Read the model definition and answer for the solid it produces. Units are mm, in the model's axes. A direction names the side the tool comes from. Give positions to 0.01 mm unless a question says otherwise; leave off trailing zeros. Write each loop counter-clockwise with the first axis right and the second up, starting at its lowest first coordinate (ties: lowest second). Pieces come first, ordered by that corner, then holes. Notation, with made-up numbers: (12.5, 80) - (70.5, 80) arc R19 cw to (70.5, 86) - close; hole circle Ø9 at (-29, 56.25). An arc over 180 degrees is marked (long way). Answer as CSV lines item,"result".
```python
from build123d import *

# Parameters (mm, degrees)
SKETCH1_R               = 10
BOSS_EXTRUDE1_DEPTH     = 10
BOSS_EXTRUDE2_DEPTH     = 110
CUT_EXTRUDE2_DEPTH      = 200.025801938
CUT_EXTRUDE2_DEPTH_BACK = 110


with BuildPart() as part:
    # Sketch1 → Boss-Extrude1 (new body)
    with BuildSketch(Plane(origin=(0, 0, 0), x_dir=(1, 0, 0), z_dir=(0, 1, 0))):
        Polygon((60, 0), (0, 0), (0, 80), (140, 80), align=None)
        with Locations(Location((40, 40, 0), (0, 0, 270))):
            Circle(SKETCH1_R, mode=Mode.SUBTRACT)
    extrude(amount=BOSS_EXTRUDE1_DEPTH)

    # Sketch1_3 → Boss-Extrude2 (add)
    with BuildSketch(Plane(origin=(0, 0, 0), x_dir=(1, 0, 0), z_dir=(0, 1, 0))):
        Polygon((140, 80), (154.142135624, 65.857864376), (74.142135624, -14.142135624), (60, 0), align=None)
    extrude(amount=BOSS_EXTRUDE2_DEPTH)

    # Sketch2 → Cut-Extrude2 (cut, two sides: drawn at the far end of the back side and taken through both)
    with BuildSketch(Plane(origin=(44.142135624, 0, 44.142135624), x_dir=(0.7071067811865461, 0, -0.707106781186549), z_dir=(0.707106781186549, 0, 0.7071067811865461)).offset(-CUT_EXTRUDE2_DEPTH_BACK)):
        with BuildLine():
            Line((42.426406871, 110), (42.426406871, 92.625413423))
            ThreePointArc((42.426406871, 92.625413423), (66.915884537, 104.857221881), (93.802749132, 110))
            Line((93.802749132, 110), (42.426406871, 110))
        make_face()
        with BuildLine():
            Line((155.563491861, 110), (104.1871496, 110))
            ThreePointArc((104.1871496, 110), (131.074014195, 104.857221881), (155.563491861, 92.625413423))
            Line((155.563491861, 92.625413423), (155.563491861, 110))
        make_face()
        with BuildLine():
            Line((58.994949366, 80), (42.426406871, 80))
            Line((42.426406871, 80), (42.426406871, 40))
            Line((42.426406871, 40), (58.994949366, 40))
            ThreePointArc((58.994949366, 40), (78.994949366, 60), (58.994949366, 80))
        make_face()
        with BuildLine():
            Line((155.563491861, 40), (155.563491861, 80))
            Line((155.563491861, 80), (138.994949366, 80))
            ThreePointArc((138.994949366, 80), (118.994949366, 60), (138.994949366, 40))
            Line((138.994949366, 40), (155.563491861, 40))
        make_face()
    extrude(amount=CUT_EXTRUDE2_DEPTH + CUT_EXTRUDE2_DEPTH_BACK, mode=Mode.SUBTRACT)


solid = part.part
```
(1) For faces 5 (the flat face through (141, 40, -67)), 6 (the flat face through (30, 5, 0)), 7 (the flat face through (73, 40, 1)), 8 (the flat face through (55, 10, -49)), 9 (the flat face through (69, 5, -80)), determine the directions among +Z, -Z, +X, -X, +Y, -Y from which every point of the face is accessible in a straight line to the end or side of a thin tool.
Worked out:
face 5,"-Z, +X"
face 6,"+Z, -X, +Y, -Y"
face 7,"+Z, -X"
face 8,"-Z, -X, +Y"
face 9,"-Z, +X, -X, +Y, -Y"
(2) A cutting plane is placed at A-A (x = 40). Write down the section's boundary in (y, z), and give its area (3 significant figures).
Worked out:
outline,"(0, -80) - (10, -80) - (10, -50) - (0, -50) - close; (0, -30) - (10, -30) - (10, 0) - (0, 0) - close"
area,"600 mm^2"
(3) Find the intervals of material crossed by L1, parallel to X at y = 7, z = -40; L2, parallel to Y at x = 73, z = 8; L3, parallel to Y at x = 49.5, z = -27.5, in increasing order.
Worked out:
L1,"x = 0 to 30, 50 to 128.28"
L2,"y = 0 to 40, 80 to 94.94"
L3,"y = 0 to 10"
(4) A cutting plane is placed at C-C (x = 13.5). Write down the section's boundary in (y, z).
Worked out:
outline,"(0, -80) - (10, -80) - (10, 0) - (0, 0) - close"
(5) A cutting plane is placed at B-B (y = 48). Write down the section's boundary in (x, z).
Worked out:
outline,"(83.03, -23.03) - (116.97, -56.97) - (131.11, -42.83) - (97.17, -8.89) - close"
(6) Each of these flat-tipped pins is pushed along its axis until it touches: P1, Ø3, axis at y = 23, z = -40.5, coming from the +X side; P2, Ø8, axis at x = 73, z = -4.5, coming from the +Y side; P3, Ø8, axis at x = 133, z = -70, coming from the +Y side; P4, Ø16, axis at x = 40, z = -40, coming from the +Y side. Where does it stop, or does it pass through?
Worked out:
P1,"stops at x = 130.28"
P2,"stops at y = 101.71"
P3,"stops at y = 101.56"
P4,"passes through"
(7) The mould has two halves that part along Z. Classify faces 1 (the flat face through (107, 110, -33)), 2 (the flat face through (147, 86, -73)), 3 (the cylindrical face through (30.24, 4.93, -42.17)), 4 (the cylindrical face through (92.83, 59.56, -18.88)): +Z half, -Z half, draft (parallel to the pull), parting line (faces both ways), or undercut.
Worked out:
face 1,"draft"
face 2,"-Z half"
face 3,"undercut"
face 4,"+Z half"
